Can you work these out from the model? Positions are in its coordinate system, mm. A direction names the side the tool comes from. Give positions to 0.01 mm unless a question says otherwise; leave off trailing zeros. Loops run counter-clockwise (first coordinate to the right, second up) from the corner with the lowest first, then second, coordinate; pieces in that order, holes last. Notation, with made-up numbers: (-27.75, 25.5) -> (-11.75, 25.5) arc R14 cw to (-11.75, 40.5) -> close; hole circle Ø9 at (54, 13). An arc over 180 degrees is marked (long way). One line per question, with ' | ' between items.
from build123d import *
from build123d.topology import SkipClean

# Parameters (mm, degrees)
BOSS_EXTRUDE1_DEPTH = 25
SKETCH2_R           = 8
CUT_EXTRUDE1_DEPTH  = 110
CUT_EXTRUDE2_DEPTH  = 150
BOSS_EXTRUDE2_START = 21.60254038
BOSS_EXTRUDE2_DEPTH = 21.60254038
SKETCH5_R           = 13
CUT_EXTRUDE3_DEPTH  = 50
SKETCH6_R           = 13
BOSS_EXTRUDE3_DEPTH = 100
SKETCH7_R           = 5
CUT_EXTRUDE4_DEPTH  = 50
SKETCH8_R           = 13
SKETCH8_R_2         = 5
BOSS_EXTRUDE4_DEPTH = 13
CUT_EXTRUDE5_DEPTH  = 28
SKETCH10_R          = 5
BOSS_EXTRUDE5_DEPTH = 10
CIRPATTERN2_COUNT   = 2
SKETCH11_W          = 47
SKETCH11_H          = 26
BOSS_EXTRUDE6_DEPTH = 10
SKETCH12_R          = 13
BOSS_EXTRUDE7_DEPTH = 67.86279097
SCALE1_SCALE        = 3.5


with BuildPart() as part:
    # Sketch1 → Boss-Extrude1 (new, symmetric)
    with BuildSketch(Plane(origin=(0, 0, 0), x_dir=(1, 0, 0), z_dir=(0, 1, 0))):
        Polygon((86.602540378, 150), (103.923048454, 160), (114.724318643, 141.291651246), (93.073683549, 128.791651246), (158.073683549, 16.208348754), (179.724318643, 28.708348754), (190.525588833, 10), (173.205080757, 0), (45.59802172, 0), (22.79901086, 39.489045172), align=None)
    extrude(amount=BOSS_EXTRUDE1_DEPTH, both=True)

    # Sketch2 → Cut-Extrude1 (cut, symmetric)
    with BuildSketch(Plane(origin=(140.729128115, 0, -81.25), x_dir=(0.8660254037844386, 0, -0.5000000000000003), z_dir=(0.5000000000000003, 0, 0.8660254037844386))):
        Circle(SKETCH2_R)
    extrude(amount=CUT_EXTRUDE1_DEPTH, both=True, mode=Mode.SUBTRACT)

    # Sketch3 → Cut-Extrude2 (cut, symmetric)
    with BuildSketch(Plane(origin=(140.729128115, 0, -81.25), x_dir=(0.8660254037844386, 0, -0.5000000000000003), z_dir=(0.5000000000000003, 0, 0.8660254037844386))):
        with BuildLine():
            Line((0, 18), (-12.5, 18))
            Line((-12.5, 18), (-12.5, 31.312178452))
            Line((-12.5, 31.312178452), (23.905899442, 31.312178452))
            Line((23.905899442, 31.312178452), (23.905899442, -29.505210198))
            Line((23.905899442, -29.505210198), (-12.5, -29.505210198))
            Line((-12.5, -29.505210198), (-12.5, -18))
            Line((-12.5, -18), (0, -18))
            ThreePointArc((0, -18), (18, 0), (0, 18))
        make_face()
    extrude(amount=CUT_EXTRUDE2_DEPTH, both=True, mode=Mode.SUBTRACT)

    # Sketch4 → Boss-Extrude2 (add)
    with SkipClean():  # the faces are left unmerged after this step: merging them gives an invalid solid
        with BuildSketch(Plane(origin=(173.229128115, 0, -24.958348754), x_dir=(0.8660254037844386, 0, -0.5000000000000003), z_dir=(0.5000000000000003, 0, 0.8660254037844386)).offset(BOSS_EXTRUDE2_START)):
            with BuildLine():
                Line((7.5, 16.363068172), (7.5, 2.783882181))
                ThreePointArc((7.5, 2.783882181), (8, 0), (7.5, -2.783882181))
                Line((7.5, -2.783882181), (7.5, -16.363068172))
                ThreePointArc((7.5, -16.363068172), (18, 0), (7.5, 16.363068172))
            make_face()
        boss_extrude2 = extrude(amount=-BOSS_EXTRUDE2_DEPTH)

    # Mirror2: Boss-Extrude2 across plane
    with SkipClean():  # the faces are left unmerged after this step: merging them gives an invalid solid
        add(boss_extrude2.mirror(Plane(origin=(140.729128115, 0, -81.25), x_dir=(-0.8660254037844388, 0, 0.5), z_dir=(0.5000000000000003, 0, 0.8660254037844386))))

    # Sketch5 → Cut-Extrude3 (cut)
    with SkipClean():  # the faces are left unmerged after this step: merging them gives an invalid solid
        with BuildSketch(Plane(origin=(34.19851629, 0, -19.744522586), x_dir=(0.5000000000000001, 0, 0.8660254037844386), z_dir=(-0.8660254037844386, 0, 0.5000000000000001))):
            Circle(SKETCH5_R)
        extrude(amount=-CUT_EXTRUDE3_DEPTH, mode=Mode.SUBTRACT)


with BuildPart() as body_2:
    # Sketch6 → Boss-Extrude3 (new body)
    with BuildSketch(Plane(origin=(77.499786479, 0, -44.744522586), x_dir=(0.5000000000000001, 0, 0.8660254037844386), z_dir=(-0.8660254037844386, 0, 0.5000000000000001))):
        with Locations(Location((0, 0, 0), (0, 0, 180))):
            Circle(SKETCH6_R)
    extrude(amount=BOSS_EXTRUDE3_DEPTH)

    # Sketch7 → Cut-Extrude4 (cut, symmetric)
    with BuildSketch(Plane(origin=(140.729128115, 0, -81.25), x_dir=(0.8660254037844386, 0, -0.5000000000000003), z_dir=(0.5000000000000003, 0, 0.8660254037844386))):
        with Locations(Location((-162.5, 0, 0), (0, 0, 180.000000003))):
            Circle(SKETCH7_R)
    extrude(amount=CUT_EXTRUDE4_DEPTH, both=True, mode=Mode.SUBTRACT)

    # Sketch8 → Boss-Extrude4 (add, symmetric)
    with BuildSketch(Plane(origin=(140.729128115, 0, -81.25), x_dir=(0.8660254037844386, 0, -0.5000000000000003), z_dir=(0.5000000000000003, 0, 0.8660254037844386))):
        with Locations((-162.5, 0)):
            Circle(SKETCH8_R)
        with Locations((-162.5, 0)):
            Circle(SKETCH8_R_2, mode=Mode.SUBTRACT)
    extrude(amount=BOSS_EXTRUDE4_DEPTH, both=True)

    # Sketch9 → Cut-Extrude5 (cut, symmetric)
    with BuildSketch(Plane(origin=(140.729128115, 0, -81.25), x_dir=(0.8660254037844386, 0, -0.5000000000000003), z_dir=(0.5000000000000003, 0, 0.8660254037844386))):
        with BuildLine():
            Line((-162.5, 13), (-162.5, 18.834095503))
            ThreePointArc((-162.5, 18.834095503), (-181.334095503, 0), (-162.5, -18.834095503))
            Line((-162.5, -18.834095503), (-162.5, -13))
            ThreePointArc((-162.5, -13), (-175.5, 0), (-162.5, 13))
        make_face()
    extrude(amount=CUT_EXTRUDE5_DEPTH, both=True, mode=Mode.SUBTRACT)


with BuildPart() as body_2_2:
    # Sketch10 → Boss-Extrude5 (new body)
    with BuildSketch(Plane(origin=(6.75, 0, 11.691342951), x_dir=(0.8660254037844385, 0, -0.5000000000000004), z_dir=(0.5000000000000003, 0, 0.8660254037844384))):
        with BuildLine():
            Line((0, 13), (21.626254201, 13))
            Line((21.626254201, 13), (21.626254201, -13))
            Line((21.626254201, -13), (0, -13))
            ThreePointArc((0, -13), (-13, 0), (0, 13))
        make_face()
        Circle(SKETCH10_R, mode=Mode.SUBTRACT)
    extrude(amount=BOSS_EXTRUDE5_DEPTH)


with BuildPart() as cirpattern2_1:
    # CirPattern2: pattern copy
    add(body_2_2.part.rotate(Axis((0, 0, 0), (-0.8660254037844385, 0, 0.5000000000000003)), 1 * 360 / CIRPATTERN2_COUNT))


with BuildPart() as body_4:
    # Sketch11 → Boss-Extrude6 (new body)
    with BuildSketch(Plane(origin=(18.728885527, 0, -10.8131271), x_dir=(-0.5000000000000004, 0, -0.8660254037844385), z_dir=(0.8660254037844384, 0, -0.5000000000000003))):
        Rectangle(SKETCH11_W, SKETCH11_H)
    extrude(amount=-BOSS_EXTRUDE6_DEPTH)


with BuildPart() as body_5:
    # Sketch12 → Boss-Extrude7 (new body)
    with BuildSketch(Plane(origin=(18.728885527, 0, -10.8131271), x_dir=(-0.5000000000000004, 0, -0.8660254037844385), z_dir=(0.8660254037844384, 0, -0.5000000000000003))):
        with Locations(Location((0, 0, 0), (0, 0, 270))):
            Circle(SKETCH12_R)
    extrude(amount=BOSS_EXTRUDE7_DEPTH)


with BuildPart() as cirpattern2_1_1:
    add(cirpattern2_1.part)

    # Combine2: union body 4, body 5, body 2 2
    add(body_4.part)
    add(body_5.part)
    add(body_2_2.part)


with BuildPart() as cirpattern2_1_2:
    # Scale1: scaled about (0, 0, 0)
    add(cirpattern2_1_1.part.scale(SCALE1_SCALE))


solid = cirpattern2_1_2.part
Q1. If we mould it in two halves opening along Z, with no side actions, what happens to faces 4 (the face through (36.14, 0.64, -88.79)), 5 (the face through (39, 45.5, -24)), 6 (the face through (35.571, 0.637, -19.773)), 7 (the face through (-71.65, 1, -33.12))? For each: pulls with the +Z half, pulls with the -Z half, needs draft (parallel to the pull), parting line crosses it, or undercut.
Entries:
face 4: pulls with the -Z half | face 5: needs draft | face 6: undercut | face 7: pulls with the +Z half
Q2. If we section it at A-A (y = -9): Write out the boundary of the cut face in (x, z), plus the area to 3 significant figures.
Entries:
outline: (-79.75, -48.93) -> (-54.12, -63.73) -> (-36.62, -33.42) -> (-62.25, -18.62) -> close; (-28.13, -78.73) -> (24.43, -109.08) -> (43.25, -76.47) -> (248.95, -195.23) -> (293.55, -117.98) -> (87.85, 0.78) -> (106.68, 33.38) -> (54.12, 63.73) -> (36.62, 33.42) -> (58.87, 20.57) -> (11.62, -61.27) -> (-10.63, -48.42) -> close; (-15, 63.22) -> (10.63, 48.42) -> (28.13, 78.73) -> (2.5, 93.53) -> close | area: 30,800 mm²
Q3. If I drill on probe 1 along X at (y, z) = (34, -109); probe 2 along Z at (x, y) = (100, 15.5); probe 3 along Z at (x, y) = (38.5, 18.5), over which ranges is the centre line in solid material (lowest first)? Write a range as from..to.
Entries:
probe 1: 24.29..24.47, 128.32..249.27 | probe 2: -107.13..-8.34, 21.82..37.24 | probe 3: -84.7..-14.7, 32.33..72.75
Q4. For pin 1 Ø4 at (y, z) = (-1.5, 57) entering from -X; pin 2 Ø1.5 at (x, y) = (229, 12.5) entering from +Z; pin 3 Ø4 at (x, z) = (137, -129) entering from +Y, each with a flat end and sliding along its axis, tell me the tip position at first contact or that it passes through.
Entries:
pin 1: x = -7.69 | pin 2: z = -81.2 | pin 3: y = 19.27
Q5. On a 3-axis mill with a long thin cutter (end or side, diameter ignored), from which of +Z, -Z, +X, -X, +Y, -Y can I reach the whole of each face in a straight line? I mean faces 1 (the face through (-44.28, 10.65, -48.92)), 2 (the face through (38.653, -9.474, 32.243)), 3 (the face through (-8.597, 9.474, -49.596)). Say none if no direction works.
Entries:
face 1: none | face 2: -X, +Y, -Y | face 3: +Y, -Y
Q6. If we section it at B-B (y = -34.5): Write out the boundary of the cut face in (x, z), plus the area to 3 significant figures.
Entries:
outline: (-66.82, -56.4) -> (24.43, -109.08) -> (50.72, -63.54) -> (256.42, -182.3) -> (286.08, -130.92) -> (80.38, -12.16) -> (106.68, 33.38) -> (15.43, 86.06) -> (-2.07, 55.75) -> (58.87, 20.57) -> (11.62, -61.27) -> (-49.32, -26.09) -> close | area: 24,800 mm²
Q7. If we section it at C-C (y = 9.5): Write out the boundary of the cut face in (x, z).
Entries:
outline: (-79.66, -48.98) -> (-53.85, -63.88) -> (-36.35, -33.57) -> (-62.16, -18.67) -> close; (-28.4, -78.58) -> (24.43, -109.08) -> (43.3, -76.38) -> (249, -195.14) -> (293.5, -118.07) -> (87.8, 0.69) -> (106.68, 33.38) -> (53.85, 63.88) -> (36.35, 33.57) -> (58.87, 20.57) -> (11.62, -61.27) -> (-10.9, -48.27) -> close; (-14.91, 63.17) -> (10.9, 48.27) -> (28.4, 78.58) -> (2.59, 93.48) -> close
